```python
from build123d import *

# Parameters (mm, degrees)
SKETCH_2_W          = 30
SKETCH_2_H          = 60
SKETCH_2_W_2        = 20
SKETCH_2_H_2        = 40
EXTRUDE_1_DEPTH     = 5
SKETCH_3_R          = 2
CUT_EXTRUDE_1_DEPTH = 5
EXTRUDE_2_DEPTH     = 5
SKETCH_6_R          = 1.5
CUT_EXTRUDE_2_DEPTH = 5
SKETCH_7_W          = 5
SKETCH_7_H          = 10
CUT_EXTRUDE_3_DEPTH = 100
SKETCH_8_W          = 30
SKETCH_8_H          = 5
EXTRUDE_3_DEPTH     = 80
SKETCH_9_W          = 30
SKETCH_9_H          = 5
EXTRUDE_4_DEPTH     = 60
SKETCH_11_W         = 30
SKETCH_11_H         = 8
EXTRUDE_5_DEPTH     = 32
EXTRUDE_6_DEPTH     = 30
SKETCH_14_W         = 30
SKETCH_14_H         = 5
EXTRUDE_7_DEPTH     = 30
SKETCH_15_W         = 37
SKETCH_15_H         = 100
EXTRUDE_8_DEPTH     = 30
SKETCH_12_R         = 3
CUT_EXTRUDE_5_DEPTH = 50
SKETCH_16_W         = 27
SKETCH_16_H         = 100
CUT_EXTRUDE_6_DEPTH = 30
SKETCH_17_R         = 3
CUT_EXTRUDE_7_DEPTH = 30


with BuildPart() as part:
    # 草图2 → 凸台-拉伸1 (new body)
    with BuildSketch(Plane.XY):
        with Locations((10, -20)):
            Rectangle(SKETCH_2_W, SKETCH_2_H)
        with Locations((10, -20)):
            Rectangle(SKETCH_2_W_2, SKETCH_2_H_2, mode=Mode.SUBTRACT)
    extrude(amount=EXTRUDE_1_DEPTH)

    # 草图3 → 切除-拉伸1 (cut)
    with BuildSketch(Plane.XY.offset(5)):
        with Locations((15.25, 5.5)):
            Circle(SKETCH_3_R)
        with Locations((15.25, -45.5)):
            Circle(SKETCH_3_R)
        with Locations((4.75, -45.5)):
            Circle(SKETCH_3_R)
        with Locations((4.75, 5.5)):
            Circle(SKETCH_3_R)
    extrude(amount=-CUT_EXTRUDE_1_DEPTH, mode=Mode.SUBTRACT)

    # 草图5 → 凸台-拉伸2 (add)
    with BuildSketch(Plane(origin=(25, 0, 0), x_dir=(0, 0, -1), z_dir=(1, 0, 0))):
        with BuildLine():
            Line((-5, -42), (-5, -40))
            Line((-5, -40), (0, -40))
            Line((0, -40), (0, -42))
            ThreePointArc((0, -42), (0.878679656, -44.121320344), (3, -45))
            Line((3, -45), (20, -45))
            Line((20, -45), (20, -50))
            Line((20, -50), (0, -50))
            Line((0, -50), (-5, -50))
            Line((-5, -50), (-25, -50))
            Line((-25, -50), (-25, -45))
            Line((-25, -45), (-8, -45))
            ThreePointArc((-8, -45), (-5.878679656, -44.121320344), (-5, -42))
        make_face()
    extrude_2 = extrude(amount=EXTRUDE_2_DEPTH)

    # 镜向1: 凸台-拉伸2 across plane
    add(extrude_2.mirror(Plane(origin=(10, 0, 0), x_dir=(0, 0, 1), z_dir=(1, 0, 0))))

    # 草图6 → 切除-拉伸2 (cut)
    with BuildSketch(Plane(origin=(0, -45, 0), x_dir=(1, 0, 0), z_dir=(0, 1, 0))):
        with Locations(Location((-7.5, 12.5, 0), (0, 0, 270))):
            Circle(SKETCH_6_R)
        with Locations(Location((-7.5, -17.5, 0), (0, 0, 270))):
            Circle(SKETCH_6_R)
        with Locations(Location((27.5, -17.5, 0), (0, 0, 270))):
            Circle(SKETCH_6_R)
        with Locations(Location((27.5, 12.5, 0), (0, 0, 270))):
            Circle(SKETCH_6_R)
    extrude(amount=-CUT_EXTRUDE_2_DEPTH, mode=Mode.SUBTRACT)

    # 草图7 → 切除-拉伸3 (cut)
    with BuildSketch(Plane.XY.offset(25)):
        with Locations((27.5, -45)):
            Rectangle(SKETCH_7_W, SKETCH_7_H)
        with Locations((-7.5, -45)):
            Rectangle(SKETCH_7_W, SKETCH_7_H)
    extrude(amount=-CUT_EXTRUDE_3_DEPTH, mode=Mode.SUBTRACT)

    # 草图8 → 凸台-拉伸3 (add)
    with BuildSketch(Plane(origin=(0, 10, 0), x_dir=(1, 0, 0), z_dir=(0, 1, 0))):
        with Locations((10, -2.5)):
            Rectangle(SKETCH_8_W, SKETCH_8_H)
    extrude(amount=EXTRUDE_3_DEPTH)

    # 草图9 → 凸台-拉伸4 (add)
    with BuildSketch(Plane.XZ.offset(50)):
        with Locations((10, 2.5)):
            Rectangle(SKETCH_9_W, SKETCH_9_H)
    extrude(amount=EXTRUDE_4_DEPTH)

    # 草图11 → 凸台-拉伸5 (add)
    with BuildSketch(Plane.XY.offset(5)):
        with Locations((10, -106)):
            Rectangle(SKETCH_11_W, SKETCH_11_H)
        with Locations((10, 86)):
            Rectangle(SKETCH_11_W, SKETCH_11_H)
    extrude(amount=EXTRUDE_5_DEPTH)

    # 草图13 → 凸台-拉伸6 (add)
    with BuildSketch(Plane(origin=(0, -102, 0), x_dir=(1, 0, 0), z_dir=(0, 1, 0))):
        Polygon((-5, -37), (25, -37), (25, -34.408335309), (25, -32), (-5, -32), align=None)
    extrude(amount=EXTRUDE_6_DEPTH)

    # 草图14 → 凸台-拉伸7 (add)
    with BuildSketch(Plane.XZ.offset(-82)):
        with Locations((10, 34.5)):
            Rectangle(SKETCH_14_W, SKETCH_14_H)
    extrude(amount=EXTRUDE_7_DEPTH)

    # 草图15 → 凸台-拉伸8 (add)
    with BuildSketch(Plane.ZY.offset(5)):
        with Locations((18.5, -160)):
            Rectangle(SKETCH_15_W, SKETCH_15_H)
    extrude(amount=-EXTRUDE_8_DEPTH)

    # 草图12 → 切除-拉伸5 (cut)
    with BuildSketch(Plane.XY.offset(5)):
        with Locations((0, 65)):
            Circle(SKETCH_12_R)
        with Locations((20, 65)):
            Circle(SKETCH_12_R)
    extrude(amount=CUT_EXTRUDE_5_DEPTH, mode=Mode.SUBTRACT)

    # 草图16 → 切除-拉伸6 (cut)
    with BuildSketch(Plane(origin=(25, 0, 0), x_dir=(0, 0, -1), z_dir=(1, 0, 0))):
        with Locations((-18.5, -152)):
            Rectangle(SKETCH_16_W, SKETCH_16_H)
    extrude(amount=-CUT_EXTRUDE_6_DEPTH, mode=Mode.SUBTRACT)

    # 草图17 → 切除-拉伸7 (cut)
    with BuildSketch(Plane.XY.offset(37)):
        with Locations((20, -190)):
            Circle(SKETCH_17_R)
        with Locations((0, -190)):
            Circle(SKETCH_17_R)
    extrude(amount=-CUT_EXTRUDE_7_DEPTH, mode=Mode.SUBTRACT)


solid = part.part
```
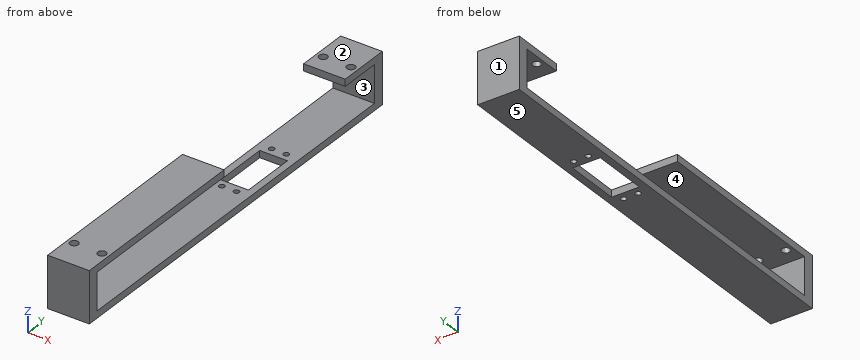
Geometry: final body of the model. Coordinates: model frame, mm. Face numbers are marked on the shaded views. A direction names the side the tool comes from. Round coordinates to 2 decimals unless told otherwise and drop trailing zeros. Write each loop counter-clockwise with the first axis right and the second up, starting at its lowest first coordinate (ties: lowest second). Pieces come first, ordered by that corner, then holes.
Item 1: Section query A-A (z = 15). Return loops of the section in (x, y), plus the area to 3 significant figures.
Item 2: Section query D-D (y = -125.5). Return loops of the section in (x, z), plus the area to 3 significant figures.
Item 3: Set-up query: the marked faces 4 and 5. Return all of +Z, -Z, +X, -X, +Y, -Y with unobstructed straight access to the full face (end or side cutting, diameter ignored); none if empty.
Item 4: Pin query (flat end, axial travel): P1, Ø2.5, axis at x = 4.75, y = -45.5, coming from the +Z side; P2, Ø9.5, axis at x = 0, y = -190, coming from the +Z side; P3, Ø6.5, axis at x = 15.25, y = -45.5, coming from the +Z side. Return the tip coordinate at first contact, or that it passes through.
Item 5: Section query C-C (y = 65). Return loops of the section in (x, z), plus the area to 3 significant figures.
Item 6: Mould query, pull axis Y, two halves, no side actions, for the marked faces 1, 2 and 3. Classes: +Y half, -Y half, draft (parallel to the pull), parting line (faces both ways), or undercut.
Item 7: Material intervals for L1, parallel to Y at x = 15.25, z = 2.25; L2, parallel to X at y = -190, z = 35.15; L3, parallel to Y at x = 0, z = 35.7, sorted ascending.
Item 8: Section query B-B (x = 9.5). Return loops of the section in (y, z), plus the area to 3 significant figures.
Completed:
1. outline: (-5, -210) - (25, -210) - (25, -202) - (-5, -202) - close; (-5, 82) - (25, 82) - (25, 90) - (-5, 90) - close
1. area: 480 mm2
2. outline: (-5, 0) - (25, 0) - (25, 5) - (-5, 5) - close; (-5, 32) - (25, 32) - (25, 37) - (-5, 37) - close
2. area: 300 mm2
3. face 4: +X, -X
3. face 5: -Z, +X, -X, +Y, -Y
4. P1: passes through
4. P2: stops at z = 37
4. P3: stops at z = 5
5. outline: (-5, 0) - (25, 0) - (25, 5) - (-5, 5) - close; (-5, 32) - (-3, 32) - (-3, 37) - (-5, 37) - close; (3, 32) - (17, 32) - (17, 37) - (3, 37) - close; (23, 32) - (25, 32) - (25, 37) - (23, 37) - close
5. area: 240 mm2
6. face 1: +Y half
6. face 2: draft
6. face 3: undercut
7. L1: y = -210 to -47.5, -43.5 to -40, 0 to 3.5, 7.5 to 90
7. L2: x = -5 to -3, 3 to 17, 23 to 25
7. L3: y = -210 to -193, -187 to -72, 52 to 62, 68 to 90
8. outline: (-210, 0) - (-40, 0) - (-40, 5) - (-202, 5) - (-202, 32) - (-72, 32) - (-72, 37) - (-210, 37) - close; (0, 0) - (90, 0) - (90, 37) - (52, 37) - (52, 32) - (82, 32) - (82, 5) - (0, 5) - close
8. area: 2,610 mm2
